Autodesk Inventor part; units mm, degrees
ref_plane "YZ Plane" through (0, 0, 0) normal (1, 0, 0) x (0, 1, 0)
ref_plane "XZ Plane" through (0, 0, 0) normal (0, 1, 0) x (-1, 0, 0)
ref_plane "XY Plane" through (0, 0, 0) normal (0, 0, 1) x (1, 0, 0)
sketch "Sketch1" plane through (0, 0, 0) normal (0, 0, 1) x (1, 0, 0)
  line L0 (0, 0) -> (0, 30)
  line L1 (0, 30) -> (5, 30)
  line L2 (5, 30) -> (2.5, 27.5)
  line L3 (2.5, 27.5) -> (2.5, 1)
  line L4 (1.5, 0) -> (0, 0)
  line L5 (2.5, 1) -> (1.5, 0)
  point P0 (2.5, 0)
  dimension "d0" = 2.5
  dimension "d2" = 5
  dimension "d3" = 135
  dimension "d4" = 30
  dimension "d6" = 1
  dimension "d7" = 1
revolve "Revolution1" add sketch "Sketch1" angle 360 about axis through (0, 0, 0) along (0, 1, 0)
sketch "Sketch2" plane through (0, 30, 0) normal (0, 1, 0) x (1, 0, 0)
  circle A0 centre (0, 0) radius 5
  line L0 (1.4802, -0.8994) -> (-0.0388, -1.7316)
  line L1 (-0.0388, -1.7316) -> (-1.519, -0.8322)
  line L2 (-1.519, -0.8322) -> (-1.4802, 0.8994)
  line L3 (-1.4802, 0.8994) -> (0.0388, 1.7316)
  line L4 (0.0388, 1.7316) -> (1.519, 0.8322)
  line L5 (1.519, 0.8322) -> (1.4802, -0.8994)
  dimension "d8" = 3
extrude "Extrusion1" cut sketch "Sketch2" against normal blind 2 contours L0 L1 L2 L3 L4 L5
properties part number "DIN7991x30"
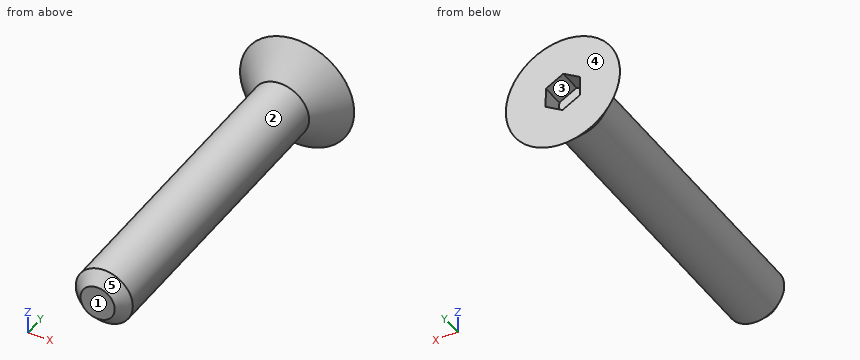
For this review, take the finished solid that the model builds, in its own axes (mm). Face numbers are marked on the shaded views. A direction names the side the tool comes from. Round coordinates to 2 decimals unless told otherwise and drop trailing zeros. Loops run counter-clockwise (first coordinate to the right, second up) from the corner with the lowest first, then second, coordinate; pieces in that order, holes last. Notation, with made-up numbers: (9.25, -9.75) - (59.25, -9.75) arc R28 ccw to (59.25, 18.25) - close; hole circle Ø9 at (71.25, -33). An arc over 180 degrees is marked (long way). Use one line per item in the form item = value.
Item 1: Clearance check with flat-ended pins moving along their axes: P1, Ø2, axis at y = 10.5, z = 1.5, coming from the +X side; P2, Ø4, axis at x = -3, y = 16, coming from the +Z side; P3, Ø4, axis at x = 0.5, z = -3.5, coming from the -Y side. State where each tip first meets the part, or that it passes through.
Answers:
P1 = 2.45
P2 = 2.29
P3 = 0.04
Item 2: Consider section A-A on z = 0. Write out the cut boundary in (x, y), then the cut area to 3 significant figures.
Answers:
outline = (-5, 30) - (-2.5, 27.5) - (-2.5, 1) - (-1.5, 0) - (1.5, 0) - (2.5, 1) - (2.5, 27.5) - (5, 30) - (1.5, 30) - (1.5, 28) - (-1.5, 28) - (-1.5, 30) - close
area = 149 mm^2
Item 3: Consider section B-B on y = 22.5. Write out the cut boundary in (x, z).
Answers:
outline = circle Ø5 at (0, 0)
Item 4: Tool access review of the marked faces 1 and 2: name each direction out of +Z, -Z, +X, -X, +Y, -Y from which nothing blocks a thin tool from reaching the whole face with its end or side.
Answers:
face_1 = +Z, -Z, +X, -X, -Y
face_2 = -Y
Item 5: For line 1 (Z direction, x = -2, y = 7.5); line 2 (Y direction, x = -0.75, z = 0.75), list the stretches that pass through material, from the lowest coordinate up.
Answers:
line_1 = -1.5 to 1.5
line_2 = 0 to 28
Item 6: Mouldability with a two-part tool opening along X and no side actions: class the marked faces 3, 4 and 5 as +X half, -X half, draft (parallel to the pull), parting line (faces both ways), or undercut.
Answers:
face_3 = undercut
face_4 = draft
face_5 = parting line
